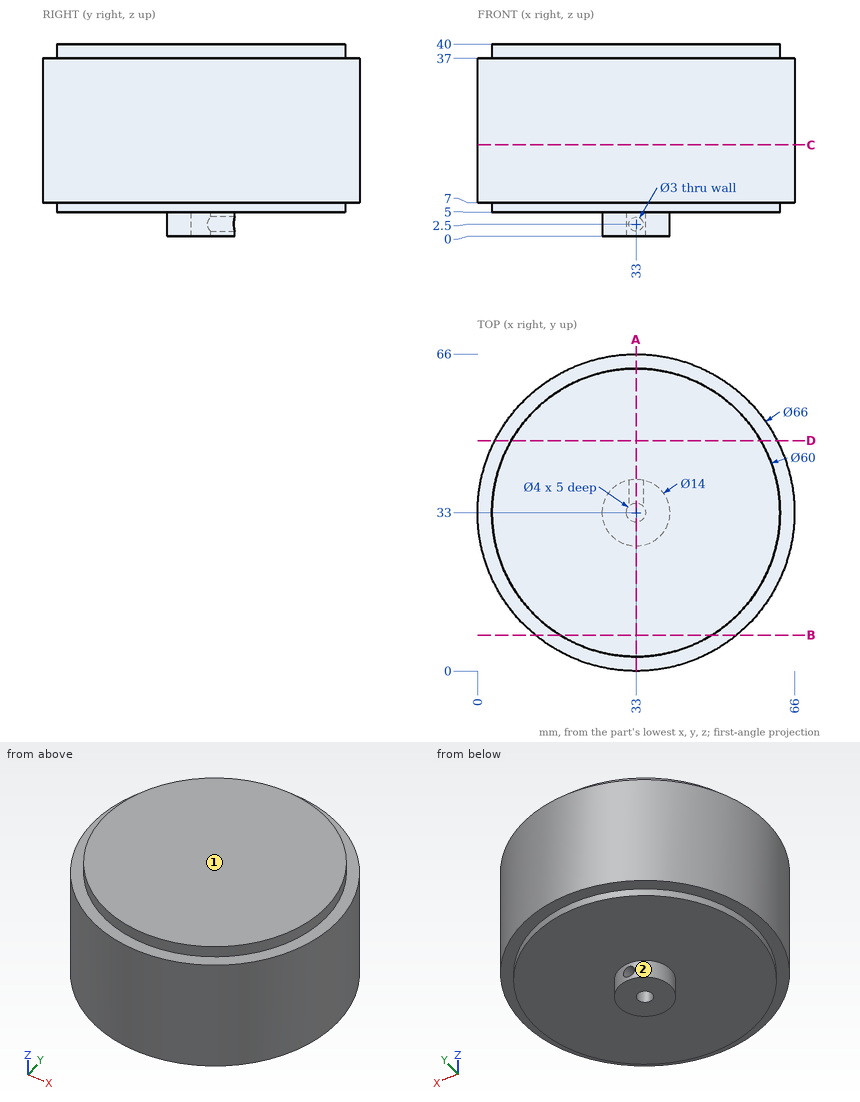
Study the drawing (mm; zero at the part's minimum x, y, z) and answer. A direction names the side the tool comes from. Round coordinates to 2 decimals unless told otherwise and drop trailing zeros. Loops run counter-clockwise (first coordinate to the right, second up) from the corner with the lowest first, then second, coordinate; pieces in that order, holes last. Notation, with made-up numbers: (57, -22.5) -> (73, -22.5) arc R17 ccw to (73, -4.5) -> close; hole circle Ø9 at (66, 42.25). An arc over 180 degrees is marked (long way). Write each question's results on one line, items separated by ' | '. Start each with the question number.
1. A tool of negligible diameter and unlimited length cuts with its end or side. For the marked faces 1 and 2, from which of +Z, -Z, +X, -X, +Y, -Y can it reach the whole face along a straight path? Write none if from no direction.
2. Find the intervals of material crossed by probe 1 along Z at (x, y) = (33, 38); probe 2 along Y at (x, z) = (33, 3.1); probe 3 along Z at (x, y) = (42, 44), in increasing order. Write a range as from..to.
3. Section A-A (x = 33) is taken. Determine the outline of the cut face in (y, z).
4. Given pin 1 Ø6 at (x, y) = (26.5, 15) entering from -Z; pin 2 Ø1.5 at (x, z) = (46.5, 24) entering from +Y; pin 3 Ø5 at (x, z) = (34.5, 7) entering from +Y, each flat-ended and moving along its own axis, determine where each tip first touches the part or whether it passes through.
5. Section D-D (y = 48) is taken. Determine the outline of the cut face in (x, z), plus the area to 3 significant figures.
6. Section B-B (y = 7.5) is taken. Determine the outline of the cut face in (x, z).
7. Section C-C (z = 19) is taken. Determine the outline of the cut face in (x, y), plus the area to 3 significant figures.
Evaluation:
1) face 1: +Z, +X, -X, +Y, -Y | face 2: -Z
2) probe 1: z = 0..1, 4..40 | probe 2: y = 26..31 | probe 3: z = 5..40
3) outline: (0, 7) -> (3, 7) -> (3, 5) -> (26, 5) -> (26, 0) -> (31, 0) -> (31, 5) -> (35, 5) -> (35, 4) -> (40, 4) -> (40, 5) -> (63, 5) -> (63, 7) -> (66, 7) -> (66, 37) -> (63, 37) -> (63, 40) -> (3, 40) -> (3, 37) -> (0, 37) -> close; (35, 0) -> (40, 0) -> (40, 1) -> (35, 1) -> close
4) pin 1: stops at z = 5 | pin 2: stops at y = 63.44 | pin 3: stops at y = 66
5) outline: (3.61, 7) -> (7.02, 7) -> (7.02, 5) -> (58.98, 5) -> (58.98, 7) -> (62.39, 7) -> (62.39, 37) -> (58.98, 37) -> (58.98, 40) -> (7.02, 40) -> (7.02, 37) -> (3.61, 37) -> close | area: 2,020 mm2
6) outline: (12.05, 7) -> (17.2, 7) -> (17.2, 5) -> (48.8, 5) -> (48.8, 7) -> (53.95, 7) -> (53.95, 37) -> (48.8, 37) -> (48.8, 40) -> (17.2, 40) -> (17.2, 37) -> (12.05, 37) -> close
7) outline: circle Ø66 at (33, 33) | area: 3,420 mm2
